Work out the finished part from the listing and answer in its coordinate system (mm). Face numbers are marked on the shaded views. A direction names the side the tool comes from. Round coordinates to 2 decimals unless told otherwise and drop trailing zeros. Write each loop counter-clockwise with the first axis right and the second up, starting at its lowest first coordinate (ties: lowest second). Pieces come first, ordered by that corner, then holes. Notation, with made-up numbers: (27.5, -3) - (60.5, -3) arc R12 cw to (60.5, 17) - close; hole circle Ø8 at (-18.75, -2). An arc over 180 degrees is marked (long way). Write item = value, one per line. Start each with the question number.
from build123d import *

# Parameters (mm, degrees)
ESQUISSE1_R                  = 9.5
BOSS_EXTRU_1_DEPTH           = 24.7
ESQUISSE2_R                  = 4
ENL_V_MAT_EXTRU_1_DEPTH      = 18
ESQUISSE3_R                  = 2.5
ENL_V_MAT_EXTRU_2_DEPTH      = 29.117432315
ESQUISSE4_R                  = 2
ENL_V_MAT_EXTRU_3_DEPTH      = 29.117432315
R_P_TITION_CIRCULAIRE1_COUNT = 2
R_P_TITION_CIRCULAIRE1_ANGLE = 90


with BuildPart() as part:
    # Esquisse1 → Boss.-Extru.1 (new body)
    with BuildSketch(Plane.XY):
        Circle(ESQUISSE1_R)
    extrude(amount=BOSS_EXTRU_1_DEPTH)

    # Esquisse2 → Enlèv. mat.-Extru.1 (cut)
    with BuildSketch(Plane.XY.offset(24.7)):
        Circle(ESQUISSE2_R)
    extrude(amount=-ENL_V_MAT_EXTRU_1_DEPTH, mode=Mode.SUBTRACT)

    # Esquisse3 → Enlèv. mat.-Extru.2 (cut, through all)
    with BuildSketch(Plane(origin=(0, 0, 0), x_dir=(-1, 0, 0), z_dir=(0, 0, -1))):
        Circle(ESQUISSE3_R)
    extrude(amount=-ENL_V_MAT_EXTRU_2_DEPTH, mode=Mode.SUBTRACT)

    # Esquisse4 → Enlèv. mat.-Extru.3 (cut, through all)
    with BuildSketch(Plane(origin=(0, 0, 0), x_dir=(1, 0, 0), z_dir=(0, 1, 0))):
        with Locations(Location((0, -4, 0), (0, 0, 270))):
            Circle(ESQUISSE4_R)
        with Locations(Location((0, -20.7, 0), (0, 0, 270))):
            Circle(ESQUISSE4_R)
    enl_v_mat_extru_3 = extrude(amount=-ENL_V_MAT_EXTRU_3_DEPTH, mode=Mode.SUBTRACT)

    # Répétition circulaire1: Enlèv. mat.-Extru.3 ×2 about axis
    r_p_tition_circulaire1_axis = Axis((0, 0, 6.7), (0, 0, -1))
    for i in range(1, R_P_TITION_CIRCULAIRE1_COUNT):
        add(enl_v_mat_extru_3.rotate(r_p_tition_circulaire1_axis, i * R_P_TITION_CIRCULAIRE1_ANGLE / (R_P_TITION_CIRCULAIRE1_COUNT - 1)), mode=Mode.SUBTRACT)


solid = part.part
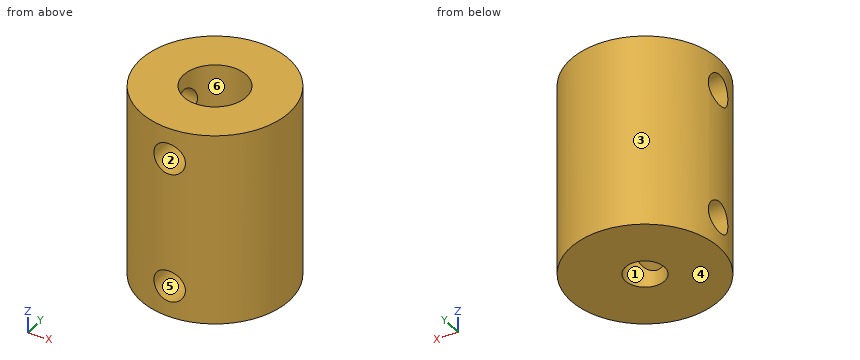
1. Each of these flat-tipped pins is pushed along its axis until it touches: pin 1 (6.5 mm diameter, centred on x = 1, y = 1.5, fed in from +Z); pin 2 (2 mm diameter, centred on y = -2.5, z = 19, fed in from +X); pin 3 (1.5 mm diameter, centred on x = -2.5, z = 5, fed in from +Y); pin 4 (3 mm diameter, centred on x = 0, z = 20.7, fed in from -Y). Where does it stop, or does it pass through?
2. Find section A-A on y = 0. Give the vertices of the cut face in (x, z).
3. Consider line 1 (Y direction, x = 0, z = 14.75); line 2 (Z direction, x = 0, y = -5.5); line 3 (Z direction, x = -5.25, y = -1). Determine where each line is inside the solid, lowest interval first.
4. Which of the six approach directions +Z, -Z, +X, -X, +Y, -Y give full straight-line access (tool end or side, diameter ignored) to the marked faces 4, 5 and 6?
5. Find section C-C on z = 4. Give the vertices of the cut face in (x, y).
6. For a pull along Y with two mould halves and no side action, classify the marked faces 1, 2 and 3 as released by +Y, released by -Y, zero draft, split by the parting line, or undercut.
7. Find section D-D on x = 3. Give the vertices of the cut face in (y, z).
Answer key:
q1.pin_1 = 24.7
q1.pin_2 = 9.38
q1.pin_3 = 9.34
q1.pin_4 = 3.71
q2.outline = (-9.5, 0) - (-2.5, 0) - (-2.5, 2) - (-9.5, 2) - close; (-9.5, 6) - (-2.5, 6) - (-2.5, 6.7) - (-4, 6.7) - (-4, 18.7) - (-9.5, 18.7) - close; (-9.5, 22.7) - (-4, 22.7) - (-4, 24.7) - (-9.5, 24.7) - close; (2.5, 0) - (9.5, 0) - (9.5, 24.7) - (4, 24.7) - (4, 6.7) - (2.5, 6.7) - close
q3.line_1 = -9.5 to -4, 4 to 9.5
q3.line_2 = 0 to 2, 6 to 18.7, 22.7 to 24.7
q3.line_3 = 0 to 2.27, 5.73 to 18.97, 22.43 to 24.7
q4.face_4 = -Z, +X, -X, +Y, -Y
q4.face_5 = -Y
q4.face_6 = +Z
q5.outline = (-9.29, -2) arc R9.5 ccw to (-2, -9.29) - (-2, -2) - close; (-9.29, 2) - (-1.5, 2) arc R2.5 cw to (2, -1.5) - (2, -9.29) arc R9.5 ccw (long way) to start
q6.face_1 = undercut
q6.face_2 = zero draft
q6.face_3 = split by the parting line
q7.outline = (-9.01, 0) - (9.01, 0) - (9.01, 24.7) - (2.65, 24.7) - (2.65, 6.7) - (-2.65, 6.7) - (-2.65, 24.7) - (-9.01, 24.7) - close
